Autodesk Inventor part; units mm, degrees
ref_plane "YZ Plane" through (0, 0, 0) normal (1, 0, 0) x (0, 1, 0)
ref_plane "XZ Plane" through (0, 0, 0) normal (0, 1, 0) x (-1, 0, 0)
ref_plane "XY Plane" through (0, 0, 0) normal (0, 0, 1) x (1, 0, 0)
sketch "Sketch1" plane through (0, 0, 0) normal (1, 0, 0) x (0, 1, 0)
  line L0 (0, 0) -> (28, 0)
  line L1 (28, 0) -> (28, -22)
  line L2 (28, -22) -> (0, -22)
  line L3 (0, -22) -> (0, 0)
  dimension "d0" = 28
  dimension "d1" = 22
extrude "Extrusion1" add sketch "Sketch1" along normal blind 5
sketch "Sketch2" plane through (0, 0, 0) normal (0, 0, 1) x (1, 0, 0)
  line L0 (0, 28) -> (5, 28)
  line L1 (0, 0) -> (5, 0)
  point P0 (2.5, 4)
  point P1 (2.5, 24)
  dimension "d4" = 4
  dimension "d5" = 4
hole "Hole1" at (2.5, 4, 0) at (2.5, 24, 0) direction (0, 0, -1) diameter 3 depth 80.45
sketch "Sketch3" plane through (5, 0, 0) normal (1, 0, 0) x (0, 0, -1)
  line L0 (22, 28) -> (0, 28)
  line L1 (0, 0) -> (22, 0)
  line L2 (0, 28) -> (0, 0)
  line L3 (11, 28) -> (11, 0)
  point P0 (4, 18)
  point P1 (4, 10)
  point P2 (18, 18)
  point P3 (18, 10)
  dimension "d13" = 10
  dimension "d14" = 10
  dimension "d15" = 4
  dimension "d16" = 4
hole "Hole2" at (5, 18, -4) at (5, 10, -4) at (5, 18, -18) at (5, 10, -18) direction (-1, 0, 0) diameter 3.2 depth 80.45
fillet "Fillet1" radius 2 4 edges at (2.5, 28, 0) (2.5, 28, -22) (2.5, 0, -22) (2.5, 0, 0)
sketch "Sketch4" plane through (5, 0, 0) normal (1, 0, 0) x (0, 0, -1)
  circle A0 centre (4, 18) radius 1.6
  circle A1 centre (18, 10) radius 1.6
  line L0 (4, 18) -> (18, 18)
  line L1 (18, 18) -> (18, 10)
  line L2 (18, 10) -> (4, 10)
  line L3 (4, 10) -> (4, 18)
  line L4 (22, 22.5) -> (0, 22.5)
  line L5 (15.75, 5.5) -> (6.25, 5.5)
  line L6 (6.25, 5.5) -> (6.25, 22.5)
  line L7 (6.25, 22.5) -> (15.75, 22.5)
  line L8 (15.75, 22.5) -> (15.75, 5.5)
  line L9 (15.75, 5.5) -> (6.25, 22.5) construction
  line L10 (6.25, 5.5) -> (15.75, 22.5) construction
  line L11 (6.25, 22.5) -> (15.75, 22.5)
  line L12 (15.75, 22.5) -> (15.75, 29.5007)
  line L13 (15.75, 29.5007) -> (6.25, 29.5007)
  line L14 (6.25, 29.5007) -> (6.25, 22.5)
  line L15 (6.25, 5.5) -> (15.75, 5.5)
  line L16 (15.75, 5.5) -> (15.75, -2.0044)
  line L17 (15.75, -2.0044) -> (6.25, -2.0044)
  line L18 (6.25, -2.0044) -> (6.25, 5.5)
  point P0 (0, 0)
  point P1 (11, 14)
  dimension "d25" = 9.5
extrude "Extrusion2" cut sketch "Sketch4" against normal blind 2 contours L6 L4 L8 L0 | L0 L8 L2 L6 | L2 L8 L5 L6
sketch "Sketch5" plane through (0, 2, -22) normal (0, 0, -1) x (-1, 0, 0)
  circle A0 centre (-2.5, 2) radius 1.5
  circle A1 centre (-2.5, 22) radius 1.5
  point P0 (0, -2)
properties part number "belt_holder_1" material "アルミニウム 6061"
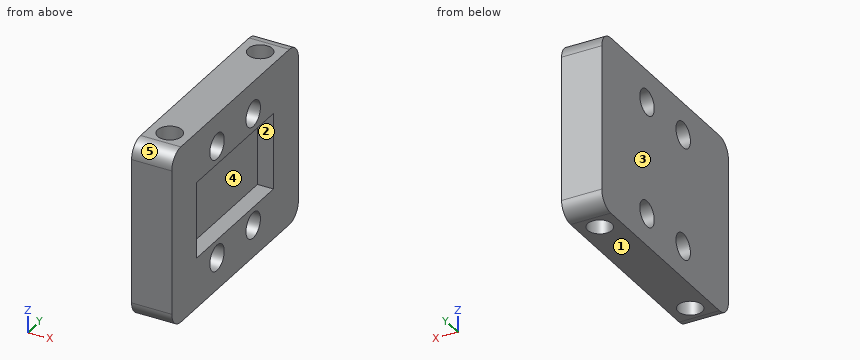
The listing builds one solid part. Answer for the finished solid, in the listing's coordinates (mm). Face numbers are marked on the shaded views. A direction names the side the tool comes from. Give positions to 0.01 mm unless a question says otherwise; leave off trailing zeros. Loops run counter-clockwise (first coordinate to the right, second up) from the corner with the lowest first, then second, coordinate; pieces in that order, holes last.
Item 1: Find the intervals of material crossed by line 1 along Z through (x, y) = (3.2, 18); line 2 along Y through (x, z) = (2.45, -18); line 3 along Y through (x, z) = (2.5, -8), in increasing order.
Derived:
line 1: z = -22 to -19.6, -16.4 to -15.75, -6.25 to -5.6, -2.4 to 0
line 2: y = 0 to 2.5, 5.5 to 8.4, 11.6 to 16.4, 19.6 to 22.5, 25.5 to 28
line 3: y = 0 to 2.5, 5.5 to 22.5, 25.5 to 28
Item 2: A tool of negligible diameter and unlimited length cuts with its end or side. For the marked faces 1 and 2, from which of +Z, -Z, +X, -X, +Y, -Y can it reach the whole face along a straight path? Write none if from no direction.
Derived:
face 1: -Z, +X, -X, +Y, -Y
face 2: +X
Item 3: A cutting plane is placed at C-C (z = -18). Give the vertices of the cut face in (x, y).
Derived:
outline: (0, 0) - (5, 0) - (5, 8.4) - (0, 8.4) - close; (0, 11.6) - (5, 11.6) - (5, 16.4) - (0, 16.4) - close; (0, 19.6) - (5, 19.6) - (5, 28) - (0, 28) - close; hole circle Ø3 at (2.5, 4); hole circle Ø3 at (2.5, 24)
Item 4: Determine the mould class of the marked faces 3, 4 and 5 for opening direction Z: +Z half, -Z half, draft (parallel to the pull), parting line (faces both ways), or undercut.
Derived:
face 3: draft
face 4: undercut
face 5: +Z half
Item 5: A cutting plane is placed at B-B (y = 24). Give the vertices of the cut face in (x, z).
Derived:
outline: (0, -22) - (1, -22) - (1, 0) - (0, 0) - close; (4, -22) - (5, -22) - (5, 0) - (4, 0) - close
Item 6: A cutting plane is placed at A-A (x = 2.5). Give the vertices of the cut face in (y, z).
Derived:
outline: (0, -20) arc R2 ccw to (2, -22) - (2.5, -22) - (2.5, 0) - (2, 0) arc R2 ccw to (0, -2) - close; (5.5, -22) - (22.5, -22) - (22.5, 0) - (5.5, 0) - close; (25.5, -22) - (26, -22) arc R2 ccw to (28, -20) - (28, -2) arc R2 ccw to (26, 0) - (25.5, 0) - close; hole circle Ø3.2 at (10, -18); hole circle Ø3.2 at (10, -4); hole circle Ø3.2 at (18, -18); hole circle Ø3.2 at (18, -4)
Item 7: A cutting plane is placed at D-D (z = -13.75). Give the vertices of the cut face in (x, y), then the cut area to 3 significant figures.
Derived:
outline: (0, 0) - (5, 0) - (5, 5.5) - (3, 5.5) - (3, 22.5) - (5, 22.5) - (5, 28) - (0, 28) - close; hole circle Ø3 at (2.5, 4); hole circle Ø3 at (2.5, 24)
area: 91.9 mm2
Item 8: This flat-tipped pin is pushed along its axis until it touches: pin 1 Ø6 at (y, z) = (10.5, -12) entering from +X. Where does it stop, or does it pass through?
Derived:
pin 1: stops at x = 3
